Input: part model. Units: mm. Frame: model coordinates. A direction names the side the tool comes from. Give positions to 0.01 mm unless a question says otherwise; leave off trailing zeros. Write each loop counter-clockwise with the first axis right and the second up, starting at its lowest first coordinate (ties: lowest second). Pieces come first, ordered by that corner, then holes. Notation, with made-up numbers: (0, 64) - (51, 64) arc R33 cw to (51, 93) - close; hole circle Ø11 at (13.5, -17). An arc over 180 degrees is marked (long way). Use a Markdown table: item, result. Add a question column.
1. Section query B-B, the plane z = 0. Return loops of the section in (x, y).
2. Set-up query: faces 4 (the flat face through (0, -2, -3)), 5 (the cylindrical face through (-1.37, 25.41, 1.04)), 6 (the flat face through (0, -2, 3)). Return all of +Z, -Z, +X, -X, +Y, -Y with unobstructed straight access to the full face (end or side cutting, diameter ignored); none if empty.
3. Pin query (flat end, axial travel): pin 1 (5 mm diameter, centred on x = 6.5, y = 12.5, fed in from -Z); pin 2 (2 mm diameter, centred on x = 4.5, z = 1.5, fed in from +Y); pin 3 (2.5 mm diameter, centred on x = -4.5, y = -3.5, fed in from +Z); pin 4 (10.5 mm diameter, centred on x = -3.5, y = 18, fed in from +Z). Return the tip coordinate at first contact, or that it passes through.
4. Section query D-D, the plane x = 7.5. Return loops of the section in (y, z).
5. Section query A-A, the plane x = 0. Return loops of the section in (y, z), plus the area to 3 significant figures.
6. Mould query, pull axis Y, two halves, no side actions, for faces 1 (the cylindrical face through (0, 29, 0)), 2 (the flat face through (-5, 6, -1.5)), 3 (the flat face through (-14, 7, 0)). Classes: released by +Y, released by -Y, zero draft, split by the parting line, or undercut.
7. Section query C-C, the plane y = 17.5. Return loops of the section in (x, z), plus the area to 3 significant figures.
8. Material intervals for probe 1 along Y at (x, z) = (0, 1.75); probe 2 along Y at (x, z) = (0, -2.15); probe 3 along Z at (x, y) = (-10, -1), sorted ascending.
```python
from build123d import *

# Parameters (mm, degrees)
BOSS_EXTRUDE1_DEPTH = 5
SKETCH2_W           = 28
SKETCH2_H           = 7
BOSS_EXTRUDE2_DEPTH = 29
CUT_EXTRUDE1_DEPTH  = 7
SKETCH4_R           = 10.5
CUT_EXTRUDE2_DEPTH  = 5
SKETCH5_R           = 9.5
CUT_EXTRUDE3_DEPTH  = 2


with BuildPart() as part:
    # Sketch1 → Boss-Extrude1 (new body)
    with BuildSketch(Plane(origin=(0, 0, 0), x_dir=(1, 0, 0), z_dir=(0, 1, 0))):
        with BuildLine():
            Line((-10.5, 3), (10.5, 3))
            ThreePointArc((10.5, 3), (13.5, 0), (10.5, -3))
            Line((10.5, -3), (-10.5, -3))
            ThreePointArc((-10.5, -3), (-13.5, 0), (-10.5, 3))
        make_face()
    extrude(amount=-BOSS_EXTRUDE1_DEPTH)

    # Sketch2 → Boss-Extrude2 (add)
    with BuildSketch(Plane(origin=(0, 0, 0), x_dir=(1, 0, 0), z_dir=(0, 1, 0))):
        Rectangle(SKETCH2_W, SKETCH2_H)
    extrude(amount=BOSS_EXTRUDE2_DEPTH)

    # Sketch3 → Cut-Extrude1 (cut)
    with BuildSketch(Plane.XY.offset(3.5)):
        with BuildLine():
            Line((-14, 15), (-14, 33.512664493))
            Line((-14, 33.512664493), (14, 33.512664493))
            Line((14, 33.512664493), (14, 15))
            ThreePointArc((14, 15), (0, 29), (-14, 15))
        make_face()
    extrude(amount=-CUT_EXTRUDE1_DEPTH, mode=Mode.SUBTRACT)

    # Sketch4 → Cut-Extrude2 (cut)
    with BuildSketch(Plane.XY.offset(3.5)):
        with Locations((0, 15)):
            Circle(SKETCH4_R)
    extrude(amount=-CUT_EXTRUDE2_DEPTH, mode=Mode.SUBTRACT)

    # Sketch5 → Cut-Extrude3 (cut)
    with BuildSketch(Plane.XY.offset(-1.5)):
        with Locations((0, 15)):
            Circle(SKETCH5_R)
    extrude(amount=-CUT_EXTRUDE3_DEPTH, mode=Mode.SUBTRACT)


solid = part.part
```
Result sheet:
| question | item | result |
|---|---|---|
| 1 | outline | (-14, 0) - (-13.5, 0) - (-13.5, -5) - (13.5, -5) - (13.5, 0) - (14, 0) - (14, 15) arc R14 ccw to (-14, 15) - close; hole circle Ø21 at (0, 15) |
| 2 | face 4 | -Z, +X, -X, -Y |
| 2 | face 5 | +Z |
| 2 | face 6 | +Z, +X, -X, -Y |
| 3 | pin 1 | passes through |
| 3 | pin 2 | stops at y = 28.56 |
| 3 | pin 3 | stops at z = 3 |
| 3 | pin 4 | stops at z = -1.5 |
| 4 | outline | (-5, -3) - (0, -3) - (0, -3.5) - (9.17, -3.5) - (9.17, -1.5) - (7.65, -1.5) - (7.65, 3.5) - (0, 3.5) - (0, 3) - (-5, 3) - close; (20.83, -3.5) - (26.82, -3.5) - (26.82, 3.5) - (22.35, 3.5) - (22.35, -1.5) - (20.83, -1.5) - close |
| 5 | outline | (-5, -3) - (0, -3) - (0, -3.5) - (5.5, -3.5) - (5.5, -1.5) - (4.5, -1.5) - (4.5, 3.5) - (0, 3.5) - (0, 3) - (-5, 3) - close; (24.5, -3.5) - (29, -3.5) - (29, 3.5) - (25.5, 3.5) - (25.5, -1.5) - (24.5, -1.5) - close |
| 5 | area | 90.0 mm² |
| 6 | face 1 | released by +Y |
| 6 | face 2 | undercut |
| 6 | face 3 | zero draft |
| 7 | outline | (-13.77, -3.5) - (-9.17, -3.5) - (-9.17, -1.5) - (-10.2, -1.5) - (-10.2, 3.5) - (-13.77, 3.5) - close; (9.17, -3.5) - (13.77, -3.5) - (13.77, 3.5) - (10.2, 3.5) - (10.2, -1.5) - (9.17, -1.5) - close |
| 7 | area | 54.2 mm² |
| 8 | probe 1 | y = -5 to 4.5, 25.5 to 29 |
| 8 | probe 2 | y = -5 to 5.5, 24.5 to 29 |
| 8 | probe 3 | z = -3 to 3 |
